Geometry check sheet. Reference: the model listing, model coordinates, mm. A direction names the side the tool comes from. Round coordinates to 2 decimals unless told otherwise and drop trailing zeros. Order: outer loops, then holes, each group sorted by start corner. A loop starts at its lowest first (then second) coordinate and runs counter-clockwise, first axis right, second up. Notation, with made-up numbers: (89.25, 72) - (122.25, 72) arc R20 ccw to (122.25, 93) - close; hole circle Ø11 at (44.25, 6.25). An arc over 180 degrees is marked (long way). One line per question, with ' | ' between items. Start each with the question number.
Q1. Gauge pin test, flat ends, axial feed: P1, Ø2, axis at x = 2, y = 15.5, coming from the -Z side; P2, Ø5, axis at y = 3.5, z = 21.5, coming from the -X side; P3, Ø14, axis at x = 8, z = -7.5, coming from the -Y side; P4, Ø22, axis at x = 1, z = 6.5, coming from the +Y side. Record the tip position at first contact, or that the pin passes through.
Q2. Sectioned sample at D-D, the plane y = 1. Enter the section's corners in (x, z).
Q3. Material ranges on line 1 along Z through (x, y) = (0, 17.25); line 2 along Z through (x, y) = (0, 12.75) (3 decimals), recorded low to high.
Q4. Tool access check on faces 4 (the face through (-5.093, 10.797, 22.936)), 5 (the face through (21.6, 17.3, -9)), 6 (the face through (-7, 16.307, -26)). Record the directions out of +Z, -Z, +X, -X, +Y, -Y that give a thin tool (end or side, any length) a straight path to the whole face; none if there is none.
Q5. Sectioned sample at B-B, the plane x = 0. Enter the section's corners in (y, z) (3 decimals).
Q6. Sectioned sample at C-C, the plane y = 9. Enter the section's corners in (x, z) (3 decimals).
Q7. Sectioned sample at A-A, the plane z = 0. Enter the section's corners in (x, y) (3 decimals), then the cut area to 3 significant figures.
Q8. Mould release check, pull along X, two halves, no side actions. Record for faces 1 (the face through (0, 0, 0)), 2 (the face through (-25.095, 17.346, -19.242)), 3 (the face through (0, 3.607, 0)): +X half, -X half, draft (parallel to the pull), parting line (faces both ways), or undercut.
Autodesk Inventor part; units mm, degrees
ref_plane "YZ Plane" through (0, 0, 0) normal (1, 0, 0) x (0, 1, 0)
ref_plane "XZ Plane" through (0, 0, 0) normal (0, 1, 0) x (-1, 0, 0)
ref_plane "XY Plane" through (0, 0, 0) normal (0, 0, 1) x (1, 0, 0)
sketch "Sketch1" plane through (0, 0, 0) normal (0, 1, 0) x (-1, 0, 0)
  circle A0 centre (0, 0) radius 26.543
  dimension "d0" = 53.086
extrude "Extrusion1" add sketch "Sketch1" along normal blind 16.3068
sketch "Sketch2" plane through (0, 16.3068, 0) normal (0, 1, 0) x (1, 0, 0)
  circle A0 centre (0, 0) radius 23.495
  dimension "d3" = 46.99
extrude "Extrusion2" cut sketch "Sketch2" against normal blind 12.7
sketch "Sketch3" plane through (0, 16.3068, 0) normal (0, 1, 0) x (1, 0, 0)
  circle A0 centre (0, 0) radius 31.623
  circle A1 centre (0, 0) radius 23.401
  dimension "d6" = 63.246
extrude "Extrusion4" add sketch "Sketch3" along normal blind 2.1082
fillet "Fillet1" radius 2.032 1 edges at (26.543, 0, 0)
fillet "Fillet2" radius 1.524 1 edges at (-23.495, 3.6068, 0)
properties part number "_3DPrint"
Determined:
1) P1: stops at z = -31.59 | P2: stops at x = -18.53 | P3: stops at y = 0 | P4: stops at y = 3.61
2) outline: circle Ø52.52 at (0, 0)
3) line 1: z = -31.62 to -23.4, 23.4 to 31.62 | line 2: z = -26.543 to -23.495, 23.495 to 26.543
4) face 4: none | face 5: +Y | face 6: -Y
5) outline: (0, -24.511) arc R2.032 ccw to (2.032, -26.543) - (16.307, -26.543) - (16.307, -31.623) - (18.415, -31.623) - (18.415, -23.401) - (16.307, -23.401) - (16.307, -23.495) - (5.131, -23.495) arc R1.524 cw to (3.607, -21.971) - (3.607, 21.971) arc R1.524 cw to (5.131, 23.495) - (16.307, 23.495) - (16.307, 23.401) - (18.415, 23.401) - (18.415, 31.623) - (16.307, 31.623) - (16.307, 26.543) - (2.032, 26.543) arc R2.032 ccw to (0, 24.511) - close
6) outline: circle Ø53.086 at (0, 0); hole circle Ø46.99 at (0, 0)
7) outline: (-31.623, 16.307) - (-26.543, 16.307) - (-26.543, 2.032) arc R2.032 ccw to (-24.511, 0) - (24.511, 0) arc R2.032 ccw to (26.543, 2.032) - (26.543, 16.307) - (31.623, 16.307) - (31.623, 18.415) - (23.401, 18.415) - (23.401, 16.307) - (23.495, 16.307) - (23.495, 5.131) arc R1.524 cw to (21.971, 3.607) - (-21.971, 3.607) arc R1.524 cw to (-23.495, 5.131) - (-23.495, 16.307) - (-23.401, 16.307) - (-23.401, 18.415) - (-31.623, 18.415) - close | area: 303 mm2
8) face 1: draft | face 2: parting line | face 3: undercut
